Model file for the job. Use its own axes, mm. Face numbers are marked on the shaded views. Coordinates: 2 decimals unless noted, no trailing zeros. Write each loop counter-clockwise with the first axis right and the second up, starting at its lowest first coordinate (ties: lowest second). Pieces come first, ordered by that corner, then holes. Notation, with made-up numbers: M -38.5,21.5 L -8.5,21.5 A22 cw -8.5,41.5 Z; hole C 52,52 d3. An arc over 180 degrees is marked long. Put each result on its own line as item: value. Start each with the question number.
Q1. Cut at A-A (x = -18). Write the cut outline in (y, z).
Q2. Drill centre lines: line 1 along Y through (x, z) = (-18, 3); line 2 along X through (y, z) = (-19, 10); line 3 along Z through (x, y) = (0, 16.5) (3 decimals). Where is each one in solid material? Low to high.
Q3. Cut at C-C (y = 18). Write the cut outline in (x, z) (3 decimals), then the cut area to 3 significant figures.
Q4. Pull direction X, two halves, no side cores. Call the marked faces 1, 2, 3 and 4: pulls with the +X half, pulls with the -X half, needs draft (parallel to the pull), parting line crosses it, or undercut.
Q5. Cut at D-D (x = 0). Write the cut outline in (y, z) (3 decimals).
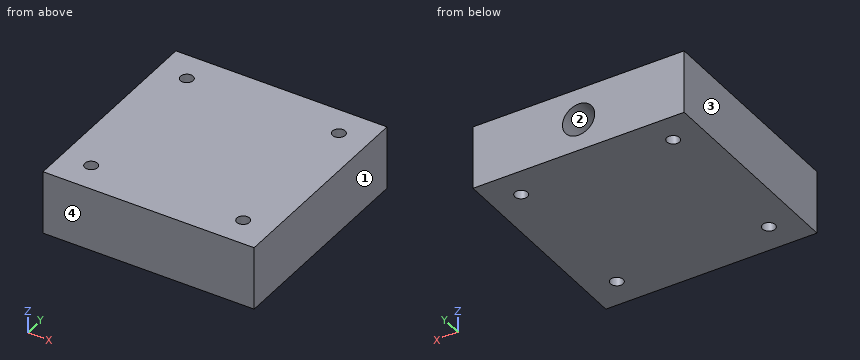
```python
from build123d import *

# Parameters (mm, degrees)
ESBO_O1_W                = 50
ESBO_O1_H                = 50
RESSALTO_EXTRUS_O1_DEPTH = 15
ESBO_O2_R                = 3.815
CORTE_EXTRUS_O1_DEPTH    = 20
ESBO_O3_R                = 1.5
CORTE_EXTRUS_O2_DEPTH    = 39.405728739


with BuildPart() as part:
    # Esboço1 → Ressalto-extrusão1 (new body)
    with BuildSketch(Plane.XY):
        Rectangle(ESBO_O1_W, ESBO_O1_H)
    extrude(amount=RESSALTO_EXTRUS_O1_DEPTH)

    # Esboço2 → Corte-extrusão1 (cut)
    with BuildSketch(Plane(origin=(0, 25, 0), x_dir=(1, 0, 0), z_dir=(0, 1, 0))):
        with Locations(Location((0, -7.5, 0), (0, 0, 180))):
            Circle(ESBO_O2_R)
    extrude(amount=-CORTE_EXTRUS_O1_DEPTH, mode=Mode.SUBTRACT)

    # Esboço3 → Corte-extrusão2 (cut, through all)
    with BuildSketch(Plane.XY.offset(15)):
        with Locations((-18, 18)):
            Circle(ESBO_O3_R)
        with Locations((-18, -18)):
            Circle(ESBO_O3_R)
        with Locations((18, 18)):
            Circle(ESBO_O3_R)
        with Locations((18, -18)):
            Circle(ESBO_O3_R)
    extrude(amount=-CORTE_EXTRUS_O2_DEPTH, mode=Mode.SUBTRACT)


solid = part.part
```
Computed values:
1. outline: M -25,0 L -19.5,0 L -19.5,15 L -25,15 Z; M -16.5,0 L 16.5,0 L 16.5,15 L -16.5,15 Z; M 19.5,0 L 25,0 L 25,15 L 19.5,15 Z
2. line 1: -25 to -19.5, -16.5 to 16.5, 19.5 to 25
2. line 2: -25 to -19.12, -16.88 to 16.88, 19.12 to 25
2. line 3: 0 to 3.685, 11.315 to 15
3. outline: M -25,0 L -19.5,0 L -19.5,15 L -25,15 Z; M -16.5,0 L 16.5,0 L 16.5,15 L -16.5,15 Z; M 19.5,0 L 25,0 L 25,15 L 19.5,15 Z; hole C 0,7.5 d7.63
3. area: 614 mm2
4. face 1: pulls with the +X half
4. face 2: undercut
4. face 3: pulls with the -X half
4. face 4: needs draft
5. outline: M -25,0 L 25,0 L 25,3.685 L 5,3.685 L 5,11.315 L 25,11.315 L 25,15 L -25,15 Z
